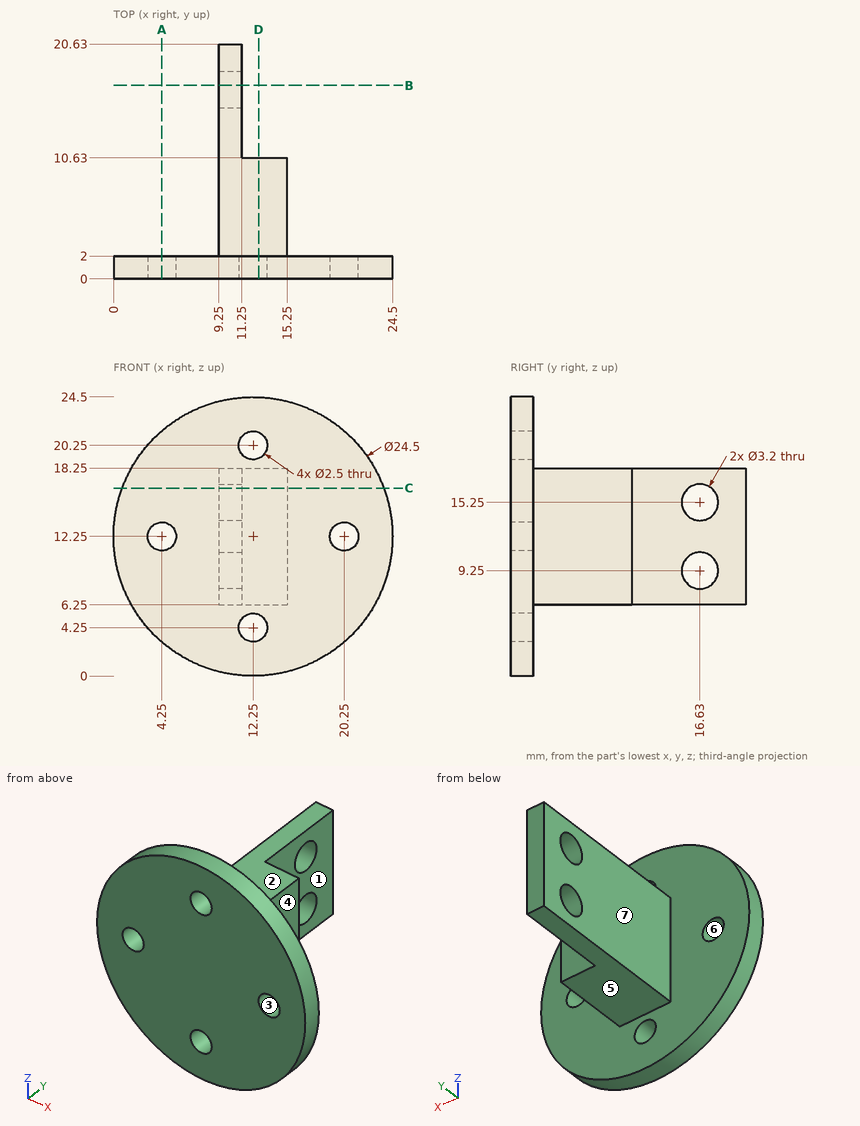
For this review, use the dimensioned drawing (mm, ordinates from the lowest corner) and the shaded views. A direction names the side the tool comes from. Give positions to 0.01 mm unless a question says otherwise; leave off trailing zeros. Order: outer loops, then holes, each group sorted by start corner. A loop starts at its lowest first (then second) coordinate and runs counter-clockwise, first axis right, second up. Notation, with made-up numbers: (69, 56) - (80, 56) arc R17 cw to (80, 88) - close; hole circle Ø2 at (-39, -1.75). An arc over 180 degrees is marked (long way). Use a Markdown table: item, result. Add a question column.
(1) Clearance check with flat-ended pins moving along their axes: P1, Ø12, axis at y = 17, z = 8.5, coming from the +X side; P2, Ø6, axis at y = 10.5, z = 5.5, coming from the +X side; P3, Ø3.5, axis at y = 8, z = 12.5, coming from the -X side. State where each tip first meets the part, or that it passes through.
(2) Add section A-A on x = 4.25. Give the boundary of the cut face in (y, z).
(3) Mouldability with a two-part tool opening along X and no side actions: class the marked faces 4, 5, 6 and 7 as +X half, -X half, draft (parallel to the pull), parting line (faces both ways), or undercut.
(4) Add section C-C on z = 16.5. Give the boundary of the cut face in (x, y).
(5) Add section D-D on x = 12.75. Give the boundary of the cut face in (y, z), then the cut area to 3 significant figures.
(6) Add section B-B on y = 17. Give the boundary of the cut face in (x, z).
(7) Machinability: for the marked faces 1, 2 and 3, which of the approach directions +Z, -Z, +X, -X, +Y, -Y give a long, thin tool a straight path to every point of the face, cutting with its end or side? Answer none if there is none.
(8) Wall thickness on probe 1 along X at (y, z) = (0.7, 12.25); probe 2 along Y at (x, z) = (10.5, 15.25); probe 3 along X at (y, z) = (7.75, 14.25): over which ranges is each line inside the solid? List them lowest first. Write a range as [from, to].
Report:
| question | item | result |
|---|---|---|
| 1 | P1 | stops at x = 11.25 |
| 1 | P2 | stops at x = 15.25 |
| 1 | P3 | stops at x = 9.25 |
| 2 | outline | (0, 2.97) - (2, 2.97) - (2, 11) - (0, 11) - close; (0, 13.5) - (2, 13.5) - (2, 21.53) - (0, 21.53) - close |
| 3 | face 4 | +X half |
| 3 | face 5 | draft |
| 3 | face 6 | undercut |
| 3 | face 7 | -X half |
| 4 | outline | (0.76, 0) - (23.74, 0) - (23.74, 2) - (15.25, 2) - (15.25, 10.63) - (11.25, 10.63) - (11.25, 15.63) - (9.25, 15.63) - (9.25, 2) - (0.76, 2) - close; (9.25, 17.63) - (11.25, 17.63) - (11.25, 20.63) - (9.25, 20.63) - close |
| 5 | outline | (0, 0.01) - (2, 0.01) - (2, 3.1) - (0, 3.1) - close; (0, 5.4) - (2, 5.4) - (2, 6.25) - (10.63, 6.25) - (10.63, 18.25) - (2, 18.25) - (2, 19.1) - (0, 19.1) - close; (0, 21.4) - (2, 21.4) - (2, 24.49) - (0, 24.49) - close |
| 5 | area | 143 mm² |
| 6 | outline | (9.25, 6.25) - (11.25, 6.25) - (11.25, 7.69) - (9.25, 7.69) - close; (9.25, 10.81) - (11.25, 10.81) - (11.25, 13.69) - (9.25, 13.69) - close; (9.25, 16.81) - (11.25, 16.81) - (11.25, 18.25) - (9.25, 18.25) - close |
| 7 | face 1 | +Z, -Z, +X, +Y |
| 7 | face 2 | +Z, +X, -X, +Y |
| 7 | face 3 | +Y, -Y |
| 8 | probe 1 | x = [0, 3], [5.5, 19], [21.5, 24.5] |
| 8 | probe 2 | y = [0, 15.03], [18.23, 20.63] |
| 8 | probe 3 | x = [9.25, 15.25] |
